For this review, take the finished solid that the model builds, in its own axes (mm). Face numbers are marked on the shaded views. Round coordinates to 2 decimals unless told otherwise and drop trailing zeros. Loops run counter-clockwise (first coordinate to the right, second up) from the corner with the lowest first, then second, coordinate; pieces in that order, holes last.
1) Mouldability with a two-part tool opening along X and no side actions: class the marked faces 1, 2, 3 and 4 as pulls with the +X half, pulls with the -X half, needs draft (parallel to the pull), parting line crosses it, or undercut.
2) Insertion check: pin 1 (5 mm diameter, centred on x = 53.5, z = -59.5, fed in from +Y). The pin has a flat end and moves straight along its axis. Give the tip position at first contact, or say it passes through.
3) Wall thickness on L1, parallel to X at y = 11.5, z = -58; L2, parallel to Z at x = 49, y = 11.25; L3, parallel to Y at x = 51.5, z = -67: over which ranges is each line inside the solid? List them lowest first.
4) Take a section at B-B (x = -85). State the section outline as (y, z) points, then the cut area to 3 significant figures.
5) Take a section at A-A (z = -52). State the section outline as (x, y) points.
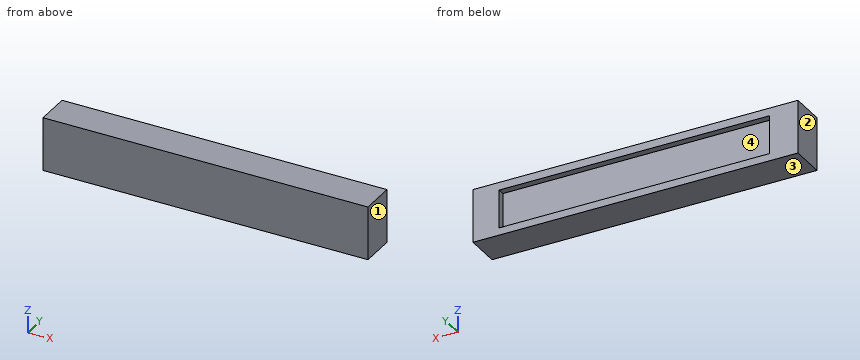
```python
from build123d import *

# Parameters (mm, degrees)
F2_W     = 233.913794
F2_H     = 38.484163
F3_DEPTH = 12.5
F4_W     = 194.459587
F4_H     = 27.622782
F5_DEPTH = 5


with BuildPart() as f3:
    # F2 (on Front) → F3 (new body, symmetric)
    with BuildSketch(Plane.XZ):
        with Locations((-0.478029, -60.131501)):
            Rectangle(F2_W, F2_H)
    extrude(amount=F3_DEPTH, both=True)

    # F4 (on face) → F5 (cut)
    with BuildSketch(Plane(origin=(0, 12.5, 0), x_dir=(-1, 0, 0), z_dir=(0, 1, 0))):
        with Locations((-0.471421, -60.297381)):
            Rectangle(F4_W, F4_H)
    extrude(amount=-F5_DEPTH, mode=Mode.SUBTRACT)


solid = f3.part
```
Response:
1. face 1: pulls with the +X half
1. face 2: pulls with the -X half
1. face 3: needs draft
1. face 4: undercut
2. pin 1: stops at y = 7.5
3. L1: x = -117.43 to -96.76, 97.7 to 116.48
3. L2: z = -79.37 to -74.11, -46.49 to -40.89
3. L3: y = -12.5 to 7.5
4. outline: (-12.5, -79.37) - (12.5, -79.37) - (12.5, -74.11) - (7.5, -74.11) - (7.5, -46.49) - (12.5, -46.49) - (12.5, -40.89) - (-12.5, -40.89) - close
4. area: 824 mm2
5. outline: (-117.43, -12.5) - (116.48, -12.5) - (116.48, 12.5) - (97.7, 12.5) - (97.7, 7.5) - (-96.76, 7.5) - (-96.76, 12.5) - (-117.43, 12.5) - close
